from build123d import *

# Parameters (mm, degrees)
SKETCH1_R           = 13
BOSS_EXTRUDE1_DEPTH = 37
SKETCH2_R           = 5
BOSS_EXTRUDE2_DEPTH = 280
SKETCH3_R           = 5
BOSS_EXTRUDE3_DEPTH = 20
FILLET1_R           = 2


with BuildPart() as part:
    # Sketch1 → Boss-Extrude1 (new body)
    with BuildSketch(Plane.XY):
        Circle(SKETCH1_R)
    extrude(amount=-BOSS_EXTRUDE1_DEPTH)

    # Sketch2 → Boss-Extrude2 (add)
    with BuildSketch(Plane.XY):
        Circle(SKETCH2_R)
    extrude(amount=BOSS_EXTRUDE2_DEPTH)

    # Sketch3 → Boss-Extrude3 (add)
    with BuildSketch(Plane.XY.offset(280)):
        Circle(SKETCH3_R)
    extrude(amount=BOSS_EXTRUDE3_DEPTH)

    # Fillet1
    fillet1_edges = [part.edges().sort_by_distance(p)[0] for p in [
        (-13, 0, 0),
        (-13, 0, -37),
        (-5, 0, 0),
    ]]
    fillet(fillet1_edges, radius=FILLET1_R)


solid = part.part
Design review of the part built by this model. Coordinates are the model's own, in mm. A direction names the side the tool comes from. Round coordinates to 2 decimals unless told otherwise and drop trailing zeros. Loops run counter-clockwise (first coordinate to the right, second up) from the corner with the lowest first, then second, coordinate; pieces in that order, holes last. Notation, with made-up numbers: (28, -26.75) - (35, -26.75) arc R11 cw to (35, -8.75) - close; hole circle Ø6 at (78, 71.25). An arc over 180 degrees is marked (long way). One line per item, written item: value. Start each with the question number.
1) Consider section C-C on z = 58. Give the boundary of the cut face in (x, y), then the cut area to 3 significant figures.
2) For faces 1 (the cylindrical face through (-10.316, -7.91, -18.269)), 2 (the cylindrical face through (-1.08, -4.88, 148.91)), list the 3-axis set-ups (+Z, -Z, +X, -X, +Y, -Y) from which the entire face can be reached by the end or side of a thin tool; tool diameter is ignored.
3) To check wall thickness, follow L1, parallel to Z at x = 0.75, y = -9; L2, parallel to Y at x = -0.75, z = 120.5; L3, parallel to Y at x = 2.25, z = 84. State the ranges of each line that lie inside material, in increasing order. Write a range as from..to.
4) Consider section A-A on x = 0. Give the boundary of the cut face in (y, z).
5) Insertion check: pin 1 Ø6 at (x, z) = (5, 67) entering from -Y; pin 2 Ø5 at (x, z) = (-2.5, 252) entering from -Y; pin 3 Ø1.5 at (x, y) = (-10, 7.5) entering from -Z. Each pin has a flat end and moves straight along its axis. Give the tip position at first contact, or say it passes through.
Reported:
1. outline: circle Ø10 at (0, 0)
1. area: 78.5 mm^2
2. face 1: +Z, -Z
2. face 2: +Z
3. L1: z = -37..0
3. L2: y = -4.94..4.94
3. L3: y = -4.47..4.47
4. outline: (-13, -35) arc R2 ccw to (-11, -37) - (11, -37) arc R2 ccw to (13, -35) - (13, -2) arc R2 ccw to (11, 0) - (7, 0) arc R2 cw to (5, 2) - (5, 300) - (-5, 300) - (-5, 2) arc R2 cw to (-7, 0) - (-11, 0) arc R2 ccw to (-13, -2) - close
5. pin 1: stops at y = -4.58
5. pin 2: stops at y = -5
5. pin 3: stops at z = -36.85
